from build123d import *

# Parameters (mm, degrees)
SKETCH_2_R           = 3
SKETCH_2_R_2         = 1.5
SKETCH_2_R_3         = 2.5
EXTRUDE_1_DEPTH      = 3
EXTRUDE_2_DEPTH      = 196
SKETCH_5_R           = 8
CUT_EXTRUDE_1_DEPTH  = 10
SKETCH_6_R           = 4.05
CUT_EXTRUDE_2_DEPTH  = 10
SKETCH_8_R           = 40
EXTRUDE_3_DEPTH      = 3
EXTRUDE_START        = -61
EXTRUDE_4_DEPTH      = 64
EXTRUDE_5_DEPTH      = 3
EXTRUDE_START_2      = -3
EXTRUDE_14_DEPTH     = 3
EXTRUDE_15_DEPTH     = 3
SKETCH_16_R          = 40
EXTRUDE_16_DEPTH     = 3
CUT_EXTRUDE_START    = -20
CUT_EXTRUDE_5_DEPTH  = 20
CUT_EXTRUDE_6_DEPTH  = 20
CUT_EXTRUDE_7_DEPTH  = 3
FILLET_3_R           = 3
FILLET_4_R           = 3
FILLET_5_R           = 3
FILLET_6_R           = 3
SKETCH_22_R          = 7.75
CUT_EXTRUDE_8_DEPTH  = 10
SKETCH_23_R          = 4.05
CUT_EXTRUDE_9_DEPTH  = 10
CUT_EXTRUDE_10_DEPTH = 10
CUT_EXTRUDE_11_DEPTH = 10
SKETCH_26_W          = 471.047466431
SKETCH_26_H          = 304.479350924
CUT_EXTRUDE_12_DEPTH = 135


# Some blends are built 0.0001 mm under size
with BuildPart() as part:
    # Sketch 2 → Extrude 1 (new body)
    with BuildSketch(Plane(origin=(0, 0, 0), x_dir=(0, 0, -1), z_dir=(1, 0, 0))):
        with BuildLine():
            Line((138.514809283, 84.200667909), (-11.70063651, 38.25042621))
            ThreePointArc((-11.70063651, 38.25042621), (-39.560188627, -5.915359313), (0, -40))
            Line((0, -40), (16.710190716, -40))
            Line((16.710190716, -40), (156.071648789, 40.329376559))
            Line((156.071648789, 40.329376559), (156.071648789, 43.792069046))
            ThreePointArc((156.071648789, 43.792069046), (165.334026038, 71.834783727), (138.514809283, 84.200667909))
        make_face()
        Circle(SKETCH_2_R, mode=Mode.SUBTRACT)
        with Locations((145, 70)):
            Circle(SKETCH_2_R_2, mode=Mode.SUBTRACT)
        with Locations((138, 63)):
            Circle(SKETCH_2_R_2, mode=Mode.SUBTRACT)
        with Locations((145, 56)):
            Circle(SKETCH_2_R_2, mode=Mode.SUBTRACT)
        with Locations((145, 63)):
            Circle(SKETCH_2_R_3, mode=Mode.SUBTRACT)
        with Locations((152, 63)):
            Circle(SKETCH_2_R_2, mode=Mode.SUBTRACT)
    extrude_1 = extrude(amount=EXTRUDE_1_DEPTH)

    # Sketch 4 → Extrude 2 (add)
    with BuildSketch(Plane(origin=(3, 0, 0), x_dir=(0, 0, -1), z_dir=(1, 0, 0))):
        with BuildLine():
            Line((0, -40), (16.710190716, -40))
            Line((16.710190716, -40), (156.071648789, 40.329376559))
            Line((156.071648789, 40.329376559), (156.071648789, 43.792069046))
            Line((156.071648789, 43.792069046), (19.975563357, -34.655113166))
            ThreePointArc((19.975563357, -34.655113166), (10.339136167, -38.640681455), (0, -40))
        make_face()
    extrude(amount=EXTRUDE_2_DEPTH)

    # Mirror 2: Extrude 1 across plane
    add(extrude_1.mirror(Plane(origin=(101, 0, 0), x_dir=(0, 0, 1), z_dir=(1, 0, 0))))

    # Sketch 5 → Cut-Extrude 1 (cut)
    with BuildSketch(Plane(origin=(202, 0, 0), x_dir=(0, 0, -1), z_dir=(1, 0, 0))):
        Circle(SKETCH_5_R)
    extrude(amount=-CUT_EXTRUDE_1_DEPTH, mode=Mode.SUBTRACT)

    # Sketch 6 → Cut-Extrude 2 (cut)
    with BuildSketch(Plane.ZY):
        Circle(SKETCH_6_R)
    extrude(amount=-CUT_EXTRUDE_2_DEPTH, mode=Mode.SUBTRACT)

    # Sketch 9 → Extrude 4 (add)
    with BuildSketch(Plane(origin=(251, 0, 0), x_dir=(0, 0, -1), z_dir=(1, 0, 0)).offset(EXTRUDE_START)):
        with BuildLine():
            Line((0, -40), (16.710190716, -40))
            Line((16.710190716, -40), (53.747942483, -18.651059269))
            Line((53.747942483, -18.651059269), (52.249775231, -16.051925781))
            Line((52.249775231, -16.051925781), (19.975563357, -34.655113166))
            ThreePointArc((19.975563357, -34.655113166), (10.339136167, -38.640681455), (0, -40))
        make_face()
    extrude_4 = extrude(amount=EXTRUDE_4_DEPTH)

    # Sketch 10 → Extrude 5 (add)
    with BuildSketch(Plane(origin=(0, -37.254246654, -21.473730609), x_dir=(1, 0, 0), z_dir=(0, -0.8663778291595938, -0.49938908392225567))):
        Polygon((254, -37.251890328), (254, -57.251890328), (202, -87.274104325), (202, -37.251890328), align=None)
    extrude_5 = extrude(amount=-EXTRUDE_5_DEPTH)



with BuildPart() as body_2:
    # Sketch 8 → Extrude 3 (new body)
    with BuildSketch(Plane(origin=(251, 0, 0), x_dir=(0, 0, -1), z_dir=(1, 0, 0))):
        Circle(SKETCH_8_R)
    extrude(amount=EXTRUDE_3_DEPTH)


with BuildPart() as part_1:
    add(part.part)

    add(body_2.part)  # Extrude 14 merges body 2
    # Sketch 14 → Extrude 14 (add)
    with BuildSketch(Plane(origin=(254, 0, 0), x_dir=(0, 0, -1), z_dir=(1, 0, 0)).offset(EXTRUDE_START_2)):
        with BuildLine():
            Line((-11.70063651, 38.25042621), (35.679778873, 52.743886101))
            Line((35.679778873, 52.743886101), (69.577331814, -6.064144103))
            Line((69.577331814, -6.064144103), (19.975563357, -34.655113166))
            ThreePointArc((19.975563357, -34.655113166), (36.686823541, 15.939792297), (-11.70063651, 38.25042621))
        make_face()
    extrude_14 = extrude(amount=EXTRUDE_14_DEPTH)

    # Sketch 15 → Extrude 15 (add)
    with BuildSketch(Plane(origin=(88.290795719, 76.368648195, -132.490087928), x_dir=(-0.8660254037844362, 0.24969454196113006, -0.43318891457980085), z_dir=(0.5000000000000046, 0.43248363304931103, -0.7503052093278205))):
        Polygon((-191.344507397, -43), (-191.344507397, 27.878041456), (-131.300079402, 20.97393325), (-131.300079402, -43), align=None)
    extrude_15 = extrude(amount=-EXTRUDE_15_DEPTH)

    # Mirror 8: Extrude 15 across plane
    add(extrude_15.mirror(Plane(origin=(101, 0, 0), x_dir=(0, 0, 1), z_dir=(1, 0, 0))))

    # Mirror 10: Extrude 5 across plane
    add(extrude_5.mirror(Plane(origin=(101, 0, 0), x_dir=(0, 0, 1), z_dir=(1, 0, 0))))

    # Mirror 11: Extrude 4 across plane
    add(extrude_4.mirror(Plane(origin=(101, 0, 0), x_dir=(0, 0, 1), z_dir=(1, 0, 0))))

    # Mirror 12: Extrude 14 across plane
    add(extrude_14.mirror(Plane(origin=(101, 0, 0), x_dir=(0, 0, 1), z_dir=(1, 0, 0))))

    # Sketch 16 → Extrude 16 (add)
    with BuildSketch(Plane.ZY.offset(52)):
        Circle(SKETCH_16_R)
    extrude(amount=-EXTRUDE_16_DEPTH)

    # Sketch 17 → Cut-Extrude 5 (cut)
    with BuildSketch(Plane(origin=(202, 0, 0), x_dir=(0, 0, -1), z_dir=(1, 0, 0)).offset(CUT_EXTRUDE_START)):
        with BuildLine():
            Line((-11.120326036, 38.423148607), (61.739147636, 60.715331959))
            Line((61.739147636, 60.715331959), (65.138195736, 61.755085767))
            Line((65.138195736, 61.755085767), (62.037518083, 60.197696416))
            Line((62.037518083, 60.197696416), (92.586691567, 7.198687311))
            Line((92.586691567, 7.198687311), (19.975563357, -34.655113166))
            ThreePointArc((19.975563357, -34.655113166), (-36.806411031, -15.66167638), (-11.120326036, 38.423148607))
        make_face()
    extrude(amount=CUT_EXTRUDE_5_DEPTH, mode=Mode.SUBTRACT)


with BuildPart() as cut_extrude_5_piece_1:
    # of the separate pieces the step leaves, piece 1, a body of its own (cut_extrude_5_pieces)
    add(part_1.part.solids().sort_by_distance((0, 43.792069046, -156.071648789))[0])

    # Sketch 21 → Cut-Extrude 7 (cut)
    with BuildSketch(Plane(origin=(3, 0, 0), x_dir=(0, 0, -1), z_dir=(1, 0, 0))):
        with BuildLine():
            Line((92.586691567, 7.198687311), (62.037518083, 60.197696416))
            Line((62.037518083, 60.197696416), (65.138195736, 61.755085767))
            Line((65.138195736, 61.755085767), (61.739147636, 60.715331959))
            Line((61.739147636, 60.715331959), (-11.70063651, 38.25042621))
            ThreePointArc((-11.70063651, 38.25042621), (-36.686823541, -15.939792297), (19.975563357, -34.655113166))
            Line((19.975563357, -34.655113166), (92.586691567, 7.198687311))
        make_face()
    extrude(amount=-CUT_EXTRUDE_7_DEPTH, mode=Mode.SUBTRACT)

    # Fillet 3
    fillet_3_edges = [cut_extrude_5_piece_1.edges().sort_by_distance(p)[0] for p in [
        (3, 33.698191863, -77.312104825),
    ]]
    fillet(fillet_3_edges, radius=FILLET_3_R - 0.0001)  # a hair under: the kernel refuses the full size

    # Fillet 4
    fillet_4_edges = [cut_extrude_5_piece_1.edges().sort_by_distance(p)[0] for p in [
        (199, 33.698191863, -77.312104825),
    ]]
    fillet(fillet_4_edges, radius=FILLET_4_R - 0.0001)  # a hair under: the kernel refuses the full size

    # Fillet 5
    # the kernel refuses this fillet: 3 mm, written as the material it adds along each edge
    with BuildSketch(Plane(origin=(202, 65.506611814, -62.97577757), x_dir=(0, 0.49938908392225567, -0.8663778291595938), z_dir=(0, -0.8663778291595938, -0.49938908392225567))) as fillet_5_piece_1_section:
        with BuildLine():
            CenterArc((FILLET_5_R * 0.57735026919, FILLET_5_R), FILLET_5_R, 210, 60)
            Line((-FILLET_5_R * 0.288675134595, FILLET_5_R * 0.5), (0, 0))
            Line((0, 0), (FILLET_5_R * 0.57735026919, 0))
        make_face()
    fillet_5_piece_1 = extrude(amount=68.304060269, mode=Mode.PRIVATE)
    fillet_5_piece_1 = split(fillet_5_piece_1, bisect_by=Plane(origin=(202.325553984, 63.906694987, -72.171998522), z_dir=(0, -0.9562606552534866, -0.2925159127537726)), keep=Keep.TOP, mode=Mode.PRIVATE)
    fillet_5_piece_1 = split(fillet_5_piece_1, bisect_by=Plane(origin=(199.177617764, 62.412552566, -67.072312804), z_dir=(0.09892666816624703, -0.8892295154916122, -0.446636746253684)), keep=Keep.TOP, mode=Mode.PRIVATE)
    add(fillet_5_piece_1)

    # Fillet 6
    # the kernel refuses this fillet: 3 mm, written as the material it adds along each edge
    with BuildSketch(Plane(origin=(0, 6.329488355, -97.086079656), x_dir=(0, 0.49938908392225556, -0.8663778291595938), z_dir=(0, 0.8663778291595938, 0.4993890839222556))) as fillet_6_piece_1_section:
        with BuildLine():
            CenterArc((FILLET_6_R * 0.57735026919, FILLET_6_R), FILLET_6_R, 210, 60)
            Line((-FILLET_6_R * 0.288675134595, FILLET_6_R * 0.5), (0, 0))
            Line((0, 0), (FILLET_6_R * 0.57735026919, 0))
        make_face()
    fillet_6_piece_1 = extrude(amount=68.304060269, mode=Mode.PRIVATE)
    fillet_6_piece_1 = split(fillet_6_piece_1, bisect_by=Plane(origin=(-0.325553984, 63.906694987, -72.171998522), z_dir=(0, -0.9562606552534866, -0.2925159127537726)), keep=Keep.TOP, mode=Mode.PRIVATE)
    fillet_6_piece_1 = split(fillet_6_piece_1, bisect_by=Plane(origin=(2.822382236, 62.412552566, -67.072312804), z_dir=(-0.09892666816624703, -0.8892295154916122, -0.446636746253684)), keep=Keep.TOP, mode=Mode.PRIVATE)
    add(fillet_6_piece_1)

    # Sketch 22 → Cut-Extrude 8 (cut)
    with BuildSketch(Plane(origin=(254, 0, 0), x_dir=(0, 0, -1), z_dir=(1, 0, 0))):
        Circle(SKETCH_22_R)
    extrude(amount=-CUT_EXTRUDE_8_DEPTH, mode=Mode.SUBTRACT)

    # Sketch 23 → Cut-Extrude 9 (cut)
    with BuildSketch(Plane.ZY.offset(52)):
        Circle(SKETCH_23_R)
    extrude(amount=-CUT_EXTRUDE_9_DEPTH, mode=Mode.SUBTRACT)

    # Sketch 24 → Cut-Extrude 10 (cut)
    with BuildSketch(Plane(origin=(0, -34.655113166, -19.975563357), x_dir=(1, 0, 0), z_dir=(0, 0.8663778291595939, 0.4993890839222556))):
        with BuildLine():
            Line((3, 179.256683584), (3, 86.81000271))
            ThreePointArc((3, 86.81000271), (2.121320344, 84.688682367), (0, 83.81000271))
            Line((0, 83.81000271), (-49, 55.51983952))
            Line((-49, 55.51983952), (-49, -19.975563357))
            Line((-49, -19.975563357), (251, -19.975563357))
            Line((251, -19.975563357), (251, 55.51983952))
            Line((251, 55.51983952), (202, 83.81000271))
            ThreePointArc((202, 83.81000271), (199.878679656, 84.688682367), (199, 86.81000271))
            Line((199, 86.81000271), (199, 179.256683584))
            Line((199, 179.256683584), (3, 179.256683584))
        make_face()
    extrude(amount=-CUT_EXTRUDE_10_DEPTH, mode=Mode.SUBTRACT)

    # Sketch 25 → Cut-Extrude 11 (cut)
    with BuildSketch(Plane.XZ.offset(40)):
        Polygon((-49, 40), (-49, -27.969882149), (251, -27.969882149), (251, 42.699584458), align=None)
    extrude(amount=-CUT_EXTRUDE_11_DEPTH, mode=Mode.SUBTRACT)


with BuildPart() as cut_extrude_5_piece_2:
    # of the separate pieces the step leaves, piece 2, a body of its own (cut_extrude_5_pieces)
    add(part_1.part.solids().sort_by_distance((202, 60.715331959, -61.739147636))[0])

    # Sketch 18 → Cut-Extrude 6 (cut)
    with BuildSketch(Plane(origin=(0, 38.25042621, 11.70063651), x_dir=(1, 0, 0), z_dir=(0, 0.9562606552534866, 0.2925159127537726))):
        Polygon((199, 76.798918519), (202, 76.932821805), (202, 0), (199, 0), align=None)
    extrude(amount=-CUT_EXTRUDE_6_DEPTH, mode=Mode.SUBTRACT)


with BuildPart() as cut_extrude_11_piece_1:
    # of the separate pieces the step leaves, piece 1, a body of its own (cut_extrude_11_pieces)
    add(cut_extrude_5_piece_1.part.solids().sort_by_distance((-1.5, 5.897004722, -96.335774447))[0])

    # Sketch 26 → Cut-Extrude 12 (cut)
    with BuildSketch(Plane(origin=(3, 0, 0), x_dir=(0, 0, -1), z_dir=(1, 0, 0))):
        with Locations((179.814409689, 100.362016139)):
            Rectangle(SKETCH_26_W, SKETCH_26_H)
    extrude(amount=-CUT_EXTRUDE_12_DEPTH, mode=Mode.SUBTRACT)


with BuildPart() as cut_extrude_11_piece_2:
    # of the separate pieces the step leaves, piece 2, a body of its own (cut_extrude_11_pieces)
    add(cut_extrude_5_piece_1.part.solids().sort_by_distance((251, -40, 0))[0])


solid = cut_extrude_11_piece_2.part
Geometry: final body of the model. Coordinates: model frame, mm. A direction names the side the tool comes from. Give positions to 0.01 mm unless a question says otherwise; leave off trailing zeros. Order: outer loops, then holes, each group sorted by start corner. A loop starts at its lowest first (then second) coordinate and runs counter-clockwise, first axis right, second up. Notation, with made-up numbers: (-26.5, 19) -> (-12.5, 19) arc R10 ccw to (-12.5, 34) -> close; hole circle Ø6 at (84, 39). An arc over 180 degrees is marked (long way). Write each question's results on one line, items separated by ' | '.
1) Set-up query: faces 1 (the face through (252.521, 7.684, 1.009)), 2 (the face through (202, 47, -116)). Return all of +Z, -Z, +X, -X, +Y, -Y with unobstructed straight access to the full face (end or side cutting, diameter ignored); none if empty.
Geometry says:
face 1: +X, -X | face 2: -Z, +X, +Y
2) Cut plane A-A (y = 0). Output: boundary loops of the cut face in (x, z), and give its area (3 significant figures).
Geometry says:
outline: (217.95, -86.11) -> (223.95, -86.11) -> (254, -66.08) -> (254, -7.75) -> (251, -7.75) -> (251, -64.08) -> close; (251, 7.75) -> (254, 7.75) -> (254, 40) -> (251, 40) -> close | area: 395 mm²
3) Line query: line 1 along Y through (x, z) = (201.15, -145); line 2 along X through (y, z) = (10, -98); line 3 along X through (y, z) = (-12, 16). Output: solid intervals per line, ascending.
Geometry says:
line 1: y = 33.95 to 54.5, 57.5 to 60.5, 65.5 to 68.5, 71.5 to 85.17 | line 2: x = 199 to 202 | line 3: x = 251 to 254
4) Cut plane C-C (x = 231.5). Output: boundary loops of the cut face in (y, z), and give its area (3 significant figures).
Geometry says:
outline: (-3.91, -79.33) -> (-2.18, -82.33) -> (56.64, -48.43) -> (55.09, -45.33) -> close | area: 236 mm²
5) Cut plane B-B (z = -59.5). Output: boundary loops of the cut face in (x, y).
Geometry says:
outline: (206.48, 59.42) -> (251, 7.95) -> (251, -15.34) -> (254, -15.34) -> (254, 11.42) -> (211.95, 60.03) -> close
6) Cut plane D-D (z = -103.5). Output: boundary loops of the cut face in (x, y).
Geometry says:
outline: (199, 10.03) -> (202, 10.03) -> (202, 73.49) -> (199, 73.49) -> close
7) Draft query along X for faces 3 (the face through (254, 7, -16)), 4 (the face through (252.479, 45.396, -11.658)), 5 (the face through (199.9, 6.34, -94.07)). Return one class per face: released by +X, released by -X, zero draft, split by the parting line, or undercut.
Geometry says:
face 3: released by +X | face 4: zero draft | face 5: released by -X
8) First-contact query: pin 1 Ø1 at (x, y) = (232, 22.5) entering from -Z; pin 2 Ø5 at (x, y) = (218.5, 34) entering from -Z; pin 3 Ø4 at (y, z) = (70, -145) entering from -X; pin 4 Ø12 at (x, y) = (233.5, 26) entering from +Z. Flat tips, straight axial feed; report the tip coordinate or a pass-through.
Geometry says:
pin 1: stops at z = -68.21 | pin 2: stops at z = -72.34 | pin 3: stops at x = 199 | pin 4: stops at z = -55.47
